Check sheet for the drawn part. Datum: minimum x, y, z corner. Units: mm. A direction names the side the tool comes from. Round coordinates to 2 decimals unless told otherwise and drop trailing zeros. Order: outer loops, then holes, each group sorted by start corner. A loop starts at its lowest first (then second) coordinate and runs counter-clockwise, first axis right, second up. Notation, with made-up numbers: M -8,71.5 L 0,71.5 A18 ccw 0,84.5 Z; hole C 73,59.25 d3. An arc over 180 degrees is marked long. Write item = value, one per line. Start each with the question number.
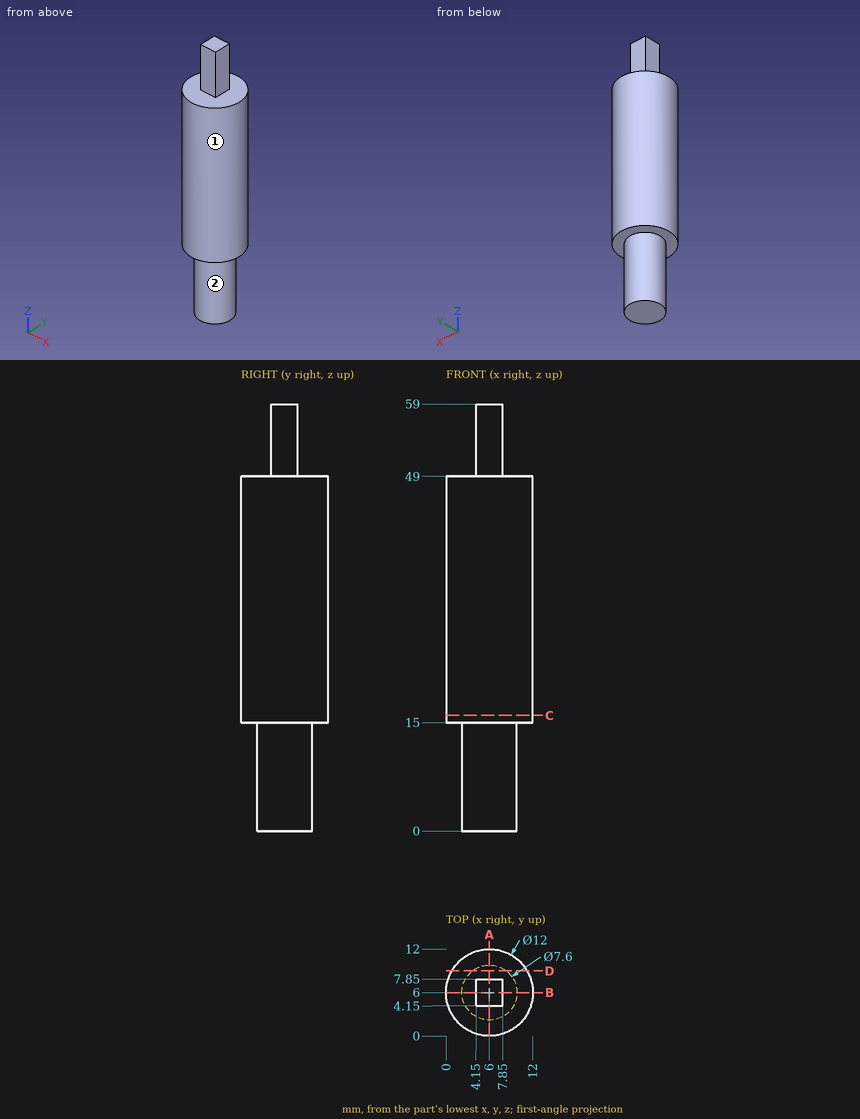
1) Access from +Z, -Z, +X, -X, +Y, -Y to the whole of each face (thin tool, end or side, straight path). Record for the marked faces 1 and 2.
2) Cross-section at C-C, the plane z = 16. Enter the section's corners in (x, y).
3) Scan lines: probe 1 along Z at (x, y) = (7.25, 1.25); probe 2 along X at (y, z) = (5.75, 31); probe 3 along Z at (x, y) = (2.5, 7). Record each from-to range of solid material in increasing order.
4) Cross-section at A-A, the plane x = 6. Enter the section's corners in (y, z).
5) Gauge pin test, flat ends, axial feed: P1, Ø6, axis at y = 10, z = 33.5, coming from the -X side; P2, Ø1, axis at x = 9.5, y = 6, coming from the -Z side; P3, Ø1.1, axis at x = 6.5, z = 55, coming from the -Y side; P4, Ø1.5, axis at x = 5.5, y = 10.5, coming from the +Z side. Record the tip position at first contact, or that the pin passes through.
6) Cross-section at D-D, the plane y = 9. Enter the section's corners in (x, z), then the cut area to 3 significant figures.
Geometry results:
q1.face_1 = +Z, -Z
q1.face_2 = -Z
q2.outline = C 6,6 d12
q3.probe_1 = 15 to 49
q3.probe_2 = 0.01 to 11.99
q3.probe_3 = 0 to 49
q4.outline = M 0,15 L 2.2,15 L 2.2,0 L 9.8,0 L 9.8,15 L 12,15 L 12,49 L 7.85,49 L 7.85,59 L 4.15,59 L 4.15,49 L 0,49 Z
q5.P1 = 0.08
q5.P2 = 0
q5.P3 = 4.15
q5.P4 = 49
q6.outline = M 0.8,15 L 3.67,15 L 3.67,0 L 8.33,0 L 8.33,15 L 11.2,15 L 11.2,49 L 0.8,49 Z
q6.area = 423 mm^2
